from build123d import *

# Parameters (mm, degrees)
SKETCH_1_R          = 1.525
SKETCH_1_R_2        = 3.025
SKETCH_1_R_3        = 1.65
EXTRUDE_1_DEPTH     = 4
SKETCH_2_R          = 1.2
CUT_EXTRUDE_1_DEPTH = 10


with BuildPart() as part:
    # 草图1 → 凸台-拉伸1 (new body)
    with BuildSketch(Plane.XY):
        with BuildLine():
            Line((15.356969673, 30.298929166), (13.674015522, 31.101791788))
            ThreePointArc((13.674015522, 31.101791788), (11.571454033, 31.125101256), (10.194791162, 29.535727958))
            ThreePointArc((10.194791162, 29.535727958), (6.381394442, 23.991783581), (0, 21.857511157))
            ThreePointArc((0, 21.857511157), (-6.773355282, 24.696305694), (-9.498676044, 31.516109427))
            ThreePointArc((-9.498676044, 31.516109427), (-9.831389744, 32.178886119), (-10.565560882, 32.28359567))
            Line((-10.565560882, 32.28359567), (-12.323298779, 31.661276982))
            ThreePointArc((-12.323298779, 31.661276982), (-13.826516548, 30.191023779), (-13.676107562, 28.09371949))
            ThreePointArc((-13.676107562, 28.09371949), (-12.45242558, 21.477080146), (-15.455594359, 15.455594359))
            ThreePointArc((-15.455594359, 15.455594359), (-22.252410678, 12.673439775), (-29.001832935, 15.568676449))
            ThreePointArc((-29.001832935, 15.568676449), (-29.705750942, 15.802066229), (-30.298929166, 15.356969673))
            Line((-30.298929166, 15.356969673), (-31.101791788, 13.674015522))
            ThreePointArc((-31.101791788, 13.674015522), (-31.125101256, 11.571454033), (-29.535727958, 10.194791162))
            ThreePointArc((-29.535727958, 10.194791162), (-23.991783581, 6.381394442), (-21.857511157, 0))
            ThreePointArc((-21.857511157, 0), (-24.696305694, -6.773355282), (-31.516109427, -9.498676044))
            ThreePointArc((-31.516109427, -9.498676044), (-32.178886119, -9.831389744), (-32.28359567, -10.565560882))
            Line((-32.28359567, -10.565560882), (-31.661276982, -12.323298779))
            ThreePointArc((-31.661276982, -12.323298779), (-30.191023779, -13.826516548), (-28.09371949, -13.676107562))
            ThreePointArc((-28.09371949, -13.676107562), (-21.477080146, -12.45242558), (-15.455594359, -15.455594359))
            ThreePointArc((-15.455594359, -15.455594359), (-12.673439775, -22.252410678), (-15.568676449, -29.001832935))
            ThreePointArc((-15.568676449, -29.001832935), (-15.802066229, -29.705750942), (-15.356969673, -30.298929166))
            Line((-15.356969673, -30.298929166), (-13.674015522, -31.101791788))
            ThreePointArc((-13.674015522, -31.101791788), (-11.571454033, -31.125101256), (-10.194791162, -29.535727958))
            ThreePointArc((-10.194791162, -29.535727958), (-6.381394442, -23.991783581), (0, -21.857511157))
            ThreePointArc((0, -21.857511157), (6.773355282, -24.696305694), (9.498676044, -31.516109427))
            ThreePointArc((9.498676044, -31.516109427), (9.831389744, -32.178886119), (10.565560882, -32.28359567))
            Line((10.565560882, -32.28359567), (12.323298779, -31.661276982))
            ThreePointArc((12.323298779, -31.661276982), (13.826516548, -30.191023779), (13.676107562, -28.09371949))
            ThreePointArc((13.676107562, -28.09371949), (12.45242558, -21.477080146), (15.455594359, -15.455594359))
            ThreePointArc((15.455594359, -15.455594359), (22.252410678, -12.673439775), (29.001832935, -15.568676449))
            ThreePointArc((29.001832935, -15.568676449), (29.705750942, -15.802066229), (30.298929166, -15.356969673))
            Line((30.298929166, -15.356969673), (31.101791788, -13.674015522))
            ThreePointArc((31.101791788, -13.674015522), (31.125101256, -11.571454033), (29.535727958, -10.194791162))
            ThreePointArc((29.535727958, -10.194791162), (23.991783581, -6.381394442), (21.857511157, 0))
            ThreePointArc((21.857511157, 0), (24.696305694, 6.773355282), (31.516109427, 9.498676044))
            ThreePointArc((31.516109427, 9.498676044), (32.178886119, 9.831389744), (32.28359567, 10.565560882))
            Line((32.28359567, 10.565560882), (31.661276982, 12.323298779))
            ThreePointArc((31.661276982, 12.323298779), (30.191023779, 13.826516548), (28.09371949, 13.676107562))
            ThreePointArc((28.09371949, 13.676107562), (21.477080146, 12.45242558), (15.455594359, 15.455594359))
            ThreePointArc((15.455594359, 15.455594359), (12.673439775, 22.252410678), (15.568676449, 29.001832935))
            ThreePointArc((15.568676449, 29.001832935), (15.802066229, 29.705750942), (15.356969673, 30.298929166))
        make_face()
        with Locations((12.597590691, 28.845398741)):
            Circle(SKETCH_1_R, mode=Mode.SUBTRACT)
        with Locations((29.304618859, 11.488935252)):
            Circle(SKETCH_1_R, mode=Mode.SUBTRACT)
        with Locations((28.845398741, -12.597590691)):
            Circle(SKETCH_1_R, mode=Mode.SUBTRACT)
        with Locations((11.488935252, -29.304618859)):
            Circle(SKETCH_1_R, mode=Mode.SUBTRACT)
        with Locations((-12.597590691, -28.845398741)):
            Circle(SKETCH_1_R, mode=Mode.SUBTRACT)
        with Locations((-29.304618859, -11.488935252)):
            Circle(SKETCH_1_R, mode=Mode.SUBTRACT)
        with Locations((-28.845398741, 12.597590691)):
            Circle(SKETCH_1_R, mode=Mode.SUBTRACT)
        with Locations((-11.488935252, 29.304618859)):
            Circle(SKETCH_1_R, mode=Mode.SUBTRACT)
        Circle(SKETCH_1_R_2, mode=Mode.SUBTRACT)
        with Locations((-8, 0)):
            Circle(SKETCH_1_R_3, mode=Mode.SUBTRACT)
        with Locations((0, 8)):
            Circle(SKETCH_1_R_3, mode=Mode.SUBTRACT)
        with Locations((8, 0)):
            Circle(SKETCH_1_R_3, mode=Mode.SUBTRACT)
        with Locations((0, -8)):
            Circle(SKETCH_1_R_3, mode=Mode.SUBTRACT)
    extrude(amount=EXTRUDE_1_DEPTH)

    # 草图2 → 切除-拉伸1 (cut)
    with BuildSketch(Plane.XY.offset(4)):
        with Locations((-6.122934918, -14.78207252)):
            Circle(SKETCH_2_R)
        with Locations((-14.78207252, 6.122934918)):
            Circle(SKETCH_2_R)
        with Locations((6.122934918, 14.78207252)):
            Circle(SKETCH_2_R)
        with Locations((14.78207252, -6.122934918)):
            Circle(SKETCH_2_R)
    extrude(amount=-CUT_EXTRUDE_1_DEPTH, mode=Mode.SUBTRACT)


solid = part.part
Build history of the part. All positions in model axes, mm. A direction names the side the tool comes from. Coordinates: 2 decimals unless noted, no trailing zeros. Write each loop counter-clockwise with the first axis right and the second up, starting at its lowest first coordinate (ties: lowest second). Pieces come first, ordered by that corner, then holes.
(1) 3-axis set-ups, long thin cutter, end or side, ignore diameter. For faces 4 (the cylindrical face through (31.137, -11.599, 1.972)), 5 (the cylindrical face through (6.46, 24.05, 1.97)): which of +Z, -Z, +X, -X, +Y, -Y reach the whole face in a straight line?
(2) Cut at C-C on y = 17. List the corners of the cut face in (x, z).
(3) Cut at A-A on y = -26.5. List the corners of the cut face in (x, z).
(4) Cut at B-B on z = 1.55. State how many separate pieces and enclosed holes the cut face has, and give its area (3 significant figures).
(5) Mould opens along X. For faces 1 (the flat face through (31.977, 11.432, 1.972)), 2 (the cylindrical face through (6.7, -24.62, 1.97)), 3 (the cylindrical face through (-13.816, 30.219, 1.972)) say: pulls with the +X half, pulls with the -X half, needs draft (parallel to the pull), parting line crosses it, or undercut.
(6) Pin check, flat tip, straight feed: pin 1 Ø5 at (x, y) = (0, 0) entering from -Z. Stop position of the tip, or through.
(7) Drill centre lines: line 1 (X direction, y = 29.5, z = 3.7); line 2 (X direction, y = -26, z = 3.5); line 3 (Y direction, x = 8, z = 3.05). Where is each one in solid material? Low to high.
(8) Cut at D-D on y = -18. List the corners of the cut face in (x, z), and give its area (3 significant figures).
Working result:
1. face 4: +Z, -Z, +X
1. face 5: +Z, -Z, +Y
2. outline: (-14.18, 0) - (14.21, 0) - (14.21, 4) - (-14.18, 4) - close
3. outline: (-13.72, 0) - (-8.77, 0) - (-8.77, 4) - (-13.72, 4) - close; (8.16, 0) - (12.96, 0) - (12.96, 4) - (8.16, 4) - close
4. separate pieces: 1
4. enclosed holes: 17
4. area: 1,950 mm2
5. face 1: pulls with the +X half
5. face 2: undercut
5. face 3: pulls with the -X half
6. pin 1: passes through
7. line 1: x = -13.98 to -13, -9.98 to -9.32, 10.18 to 11.22, 13.97 to 15.81
7. line 2: x = -13.48 to -8.41, 7.85 to 12.79
7. line 3: y = -26.23 to -1.65, 1.65 to 25.5
8. outline: (-13.64, 0) - (13.58, 0) - (13.58, 4) - (-13.64, 4) - close
8. area: 109 mm2
